The listing builds one solid part. Answer for the finished solid, in the listing's coordinates (mm). A direction names the side the tool comes from. Coordinates: 2 decimals unless noted, no trailing zeros. Write each loop counter-clockwise with the first axis right and the second up, starting at its lowest first coordinate (ties: lowest second). Pieces come first, ordered by that corner, then holes.
Autodesk Inventor part; units mm, degrees
ref_plane "Arbeitsebene2" through (-22.5, -14.565, -0.4115) normal (0, 0, -1) x (0, 1, 0)
ref_plane "Arbeitsebene3" through (-22.5, -14.565, 0) normal (0, 0, 1) x (1, 0, 0)
ref_plane "YZ Plane" through (0, 0, 0) normal (1, 0, 0) x (0, 1, 0)
ref_plane "Arbeitsebene1" through (0, 0, 6) normal (0, 0, 1) x (1, 0, 0)
sketch "Skizze3" plane through (0, 0, 6) normal (0, 0, 1) x (1, 0, 0)
  line L0 (22.5, -14.565) -> (22.5, 14.565)
  line L1 (-22.5, -14.565) -> (22.5, -14.565)
  line L2 (-22.5, 10.565) -> (-22.5, -14.565)
  line L3 (22.5, 14.565) -> (-18.5, 14.565)
  circle A0 centre (19.6, -11.465) radius 1.5
  circle A1 centre (13.06, -2.125) radius 0.65
  circle A2 centre (13.06, -4.665) radius 0.65
  circle A3 centre (13.06, 0.415) radius 0.65
  circle A4 centre (13.06, 2.955) radius 0.65
  circle A5 centre (-2.18, 5.495) radius 0.65
  circle A6 centre (13.06, 5.495) radius 0.65
  circle A7 centre (19.6, 11.535) radius 1.5
  circle A8 centre (13.06, 8.035) radius 0.65
  circle A9 centre (13.06, 10.575) radius 0.65
  circle A10 centre (-2.18, 8.035) radius 0.65
  circle A11 centre (13.06, 13.115) radius 0.65
  circle A12 centre (-2.18, 10.575) radius 0.65
  circle A13 centre (-7.26, -6.945) radius 0.5
  circle A14 centre (-2.18, -2.125) radius 0.65
  circle A15 centre (-2.18, -4.665) radius 0.65
  circle A16 centre (-12.34, -6.945) radius 0.5
  circle A17 centre (-19.4, -11.465) radius 1.5
  circle A18 centre (-7.26, -4.405) radius 0.5
  circle A19 centre (-12.34, -4.405) radius 0.5
  circle A20 centre (-2.18, 0.415) radius 0.65
  circle A21 centre (-2.18, 13.115) radius 0.65
  circle A22 centre (-2.18, 2.955) radius 0.65
  circle A23 centre (-7.26, -1.865) radius 0.5
  circle A24 centre (-12.34, -1.865) radius 0.5
  circle A25 centre (-7.26, 0.675) radius 0.5
  circle A26 centre (-12.34, 0.675) radius 0.5
  line L4 (-24.7, -16.765) -> (24.7, -16.765)
  line L5 (24.7, -16.765) -> (24.7, 16.765)
  line L6 (24.7, 16.765) -> (-24.7, 16.765)
  line L7 (-24.7, 16.765) -> (-24.7, -16.765)
  line L8 (-24.34, 2.175) -> (-10.84, 2.175)
  line L9 (-10.84, 2.175) -> (-10.84, -8.525)
  line L10 (-10.84, -8.525) -> (-24.34, -8.525)
  line L11 (-24.34, -8.525) -> (-24.34, 2.175)
  circle A27 centre (-12.34, -1.865) radius 0.5
  circle A28 centre (-12.34, -4.405) radius 0.5
  circle A29 centre (-12.34, -6.945) radius 0.5
  circle A30 centre (-12.34, 0.675) radius 0.5
  circle A31 centre (-21.39, -0.725) radius 1.5
  line L12 (24.7, 16.765) -> (-26.94, 16.765)
  line L13 (-26.94, 16.765) -> (-26.94, -16.765)
  line L14 (-26.94, -16.765) -> (24.7, -16.765)
  line L15 (24.7, -16.765) -> (24.7, 16.765)
  line L16 (-18.5, 10.565) -> (-18.5, 14.565)
  line L17 (-22.5, 10.565) -> (-18.5, 10.565)
  point P0 (0, 0)
  point P1 (-24.7, 16.765)
  dimension "d5" = 2.2
  dimension "d6" = 2.6
extrude "Extrusion2" add sketch "Skizze3" against normal blind 2 contours L1 L2 L10 L9 L8 L17 L16 L3 L0 | L10 L11 L8 L2 A31 | L2 A31 L8 L9 L10 | A31 L2 | L2 A31 | A0 | A1 | A2 | A3 | A4 | A5 | A6 | A7 | A8 | A9 | A10 | A11 | A12 | A13 | A14 | A15 | A16 | A17 | A18 | A19 | A20 | A21 | A22 | A23 | A24 | A25 | A26 | L7 L6 L5 L4 | L14 L13 L12 L7
sketch "Skizze4" plane through (0, 0, 4) normal (0, 0, -1) x (-1, 0, 0)
  line L0 (-24.7, 16.765) -> (-24.7, -16.765)
  line L1 (-24.7, -16.765) -> (26.94, -16.765)
  line L2 (26.94, -16.765) -> (26.94, 16.765)
  line L3 (26.94, 16.765) -> (-24.7, 16.765)
  line L4 (-22.7, 14.765) -> (-22.7, -14.765)
  line L5 (-22.7, -14.765) -> (24.94, -14.765)
  line L6 (24.94, -14.765) -> (24.94, 14.765)
  line L7 (24.94, 14.765) -> (-22.7, 14.765)
  point P0 (0, 0)
  dimension "d9" = 2
ref_plane "Arbeitsebene2" through (-22.5, -14.565, -0.4115) normal (0, 0, -1) x (0, 1, 0)
extrude "Extrusion3" add sketch "Skizze4" along normal up to surface (4.4115 mm away)
sketch "Skizze5" plane through (24.7, -16.765, -0.4115) normal (0, 0, -1) x (-1, 0, 0)
  line L0 (2, 31.53) -> (2, 2)
  line L1 (49.64, 31.53) -> (2, 31.53)
  line L2 (49.64, 2) -> (49.64, 31.53)
  line L3 (2, 2) -> (49.64, 2)
  line L4 (0, 0) -> (0, 33.53)
  line L5 (51.64, 0) -> (0, 0)
  line L6 (51.64, 33.53) -> (51.64, 0)
  line L7 (0, 33.53) -> (51.64, 33.53)
  line L8 (50.64, 32.53) -> (50.64, 1)
  line L9 (50.64, 1) -> (1, 1)
  line L10 (1, 1) -> (1, 32.53)
  line L11 (1, 32.53) -> (50.64, 32.53)
  point P0 (24.7, 16.765)
  dimension "d12" = 1
extrude "Extrusion4" cut sketch "Skizze5" against normal blind 2 contours L4 L7 L6 L5
sketch "Skizze6" plane through (0, 0, 4) normal (0, 0, -1) x (-1, 0, 0)
  circle A0 centre (-19.6, 11.535) radius 1.5
  circle A1 centre (-19.6, -11.465) radius 1.5
  circle A2 centre (19.4, -11.465) radius 1.5
  circle A3 centre (-19.6, -11.465) radius 1.7
  circle A4 centre (-19.6, 11.535) radius 1.7
  circle A5 centre (19.4, -11.465) radius 1.7
  line L0 (-22.7, -14.765) -> (24.94, -14.765)
  line L1 (-22.7, -14.765) -> (-16.5, -14.765)
  line L2 (-16.5, -14.765) -> (-16.5, -10.165)
  line L3 (-18.5, -8.165) -> (-22.7, -8.165)
  line L4 (-22.7, -8.165) -> (-22.7, -14.765)
  arc A6 (-16.5, -10.165) -> (-18.5, -8.165) centre (-18.5, -10.165) ccw
  line L5 (24.94, 14.765) -> (-22.7, 14.765)
  line L6 (-22.7, 14.765) -> (-16.5, 14.765)
  line L7 (-16.5, 14.765) -> (-16.5, 10.165)
  line L8 (-18.5, 8.165) -> (-22.7, 8.165)
  line L9 (-22.7, 8.165) -> (-22.7, 14.765)
  line L10 (24.94, -14.765) -> (16.3, -14.765)
  line L11 (16.3, -14.765) -> (16.3, -10.165)
  line L12 (18.3, -8.165) -> (24.94, -8.165)
  line L13 (24.94, -8.165) -> (24.94, -14.765)
  arc A7 (18.3, -8.165) -> (16.3, -10.165) centre (18.3, -10.165) ccw
  arc A8 (-18.5, 8.165) -> (-16.5, 10.165) centre (-18.5, 10.165) ccw
  line L14 (24.94, 14.765) -> (16.3, 14.765)
  line L15 (16.3, 14.765) -> (16.3, 10.165)
  line L16 (18.3, 8.165) -> (24.94, 8.165)
  line L17 (24.94, 8.165) -> (24.94, 14.765)
  arc A9 (16.3, 10.165) -> (18.3, 8.165) centre (18.3, 10.165) ccw
  point P0 (0, 0)
  point P1 (-16.5, -8.165)
  point P2 (-16.5, 8.165)
  dimension "d15" = 0.2
  dimension "d16" = 0.2
  dimension "d17" = 0.2
  dimension "d18" = 6.2
  dimension "d19" = 6.6
  dimension "d20" = 2
  dimension "d21" = 6.2
  dimension "d22" = 6.6
  dimension "d23" = 3.3
  dimension "d24" = 3.1
  dimension "d25" = 2
  dimension "d26" = 2
ref_plane "Arbeitsebene3" through (-22.5, -14.565, 0) normal (0, 0, 1) x (1, 0, 0)
extrude "Extrusion5" add sketch "Skizze6" along normal blind 2.211 contours L4 L3 A6 L2 L0 | L11 A7 L12 L13 L0 | L17 L16 A9 L15 L5 | L7 A8 L8 L9 L5
sketch "Skizze7" plane through (19.6, 11.535, 4) normal (0, 0, -1) x (-1, 0, 0)
  circle A0 centre (0, 0) radius 1.7
  circle A1 centre (0, -23) radius 1.7
  circle A2 centre (39, -23) radius 1.7
  point P0 (19.6, -11.535)
extrude "Extrusion6" cut sketch "Skizze7" against normal up to surface (2 mm away)
sketch "Skizze8" plane through (0, 0, 6) normal (0, 0, 1) x (1, 0, 0)
  circle A0 centre (19.6, -11.465) radius 1.7
  circle A1 centre (19.6, 11.535) radius 1.7
  circle A2 centre (-19.4, -11.465) radius 1.7
  line L0 (24.7, -16.765) -> (24.7, 16.765)
  line L1 (24.7, 16.765) -> (-26.94, 16.765)
  line L2 (-26.94, 16.765) -> (-26.94, -16.765)
  line L3 (-26.94, -16.765) -> (24.7, -16.765)
  line L4 (16.75, -9.8196) -> (19.6, -8.1741)
  line L5 (19.6, -8.1741) -> (22.45, -9.8196)
  line L6 (22.45, -9.8196) -> (22.45, -13.1104)
  line L7 (22.45, -13.1104) -> (19.6, -14.7559)
  line L8 (19.6, -14.7559) -> (16.75, -13.1104)
  line L9 (16.75, -13.1104) -> (16.75, -9.8196)
  line L10 (16.75, 13.1804) -> (19.6, 14.8259)
  line L11 (19.6, 14.8259) -> (22.45, 13.1804)
  line L12 (22.45, 13.1804) -> (22.45, 9.8896)
  line L13 (22.45, 9.8896) -> (19.6, 8.2441)
  line L14 (19.6, 8.2441) -> (16.75, 9.8896)
  line L15 (16.75, 9.8896) -> (16.75, 13.1804)
  line L16 (-22.25, -9.8196) -> (-19.4, -8.1741)
  line L17 (-19.4, -8.1741) -> (-16.55, -9.8196)
  line L18 (-16.55, -9.8196) -> (-16.55, -13.1104)
  line L19 (-16.55, -13.1104) -> (-19.4, -14.7559)
  line L20 (-19.4, -14.7559) -> (-22.25, -13.1104)
  line L21 (-22.25, -13.1104) -> (-22.25, -9.8196)
  line L22 (24.7, -16.765) -> (24.7, 16.765)
  point P0 (0, 0)
  dimension "d31" = 5.7
  dimension "d32" = 5.7
  dimension "d33" = 5.7
extrude "Extrusion7" cut sketch "Skizze8" against normal blind 2.6 contours A0 | A1 | A2 | L4 L5 L6 L7 L8 L9 | L10 L11 L12 L13 L14 L15 | L16 L17 L18 L19 L20 L21
fillet "Rundung1" radius 2 4 edges at (24.7, -16.765, 3.7943) (-26.94, -16.765, 3.7943) (-26.94, 16.765, 5) (24.7, 16.765, 3.7943)
fillet "Rundung2" radius 1 4 edges at (-25.94, -15.765, 0.5885) (-25.94, 15.765, 0.5885) (23.7, 15.765, 0.5885) (23.7, -15.765, 0.5885)
sketch "Skizze9" plane through (0, 0, 1.789) normal (0, 0, -1) x (-1, 0, 0)
  line L0 (24.94, 14.765) -> (24.94, 8.165)
  line L1 (24.94, 14.765) -> (21.64, 14.765)
  line L2 (21.64, 14.765) -> (21.64, 11.465)
  line L3 (21.64, 11.465) -> (24.94, 11.465)
  line L4 (24.94, 11.465) -> (24.94, 14.765)
  circle A0 centre (23.29, 13.115) radius 1.65
  point P0 (0, 0)
  dimension "d38" = 3.3
  dimension "d39" = 3.3
extrude "Extrusion8" cut sketch "Skizze9" against normal blind 10 contours A0
sketch "Skizze10" plane through (0, 0, 6) normal (0, 0, 1) x (1, 0, 0)
  arc A0 (-24.94, 13.115) -> (-23.29, 14.765) centre (-23.29, 13.115) ccw
  line L0 (-20.44, 11.4696) -> (-23.29, 9.8241)
  line L1 (-23.29, 9.8241) -> (-26.14, 11.4696)
  line L2 (-26.14, 11.4696) -> (-26.14, 14.7604)
  line L3 (-26.14, 14.7604) -> (-23.29, 16.4059)
  line L4 (-23.29, 16.4059) -> (-20.44, 14.7604)
  line L5 (-20.44, 14.7604) -> (-20.44, 11.4696)
  line L6 (-26.94, 14.765) -> (-26.94, -14.765)
  point P0 (0, 0)
  point P1 (-26.14, 13.115)
  dimension "d42" = 5.7
extrude "Extrusion9" cut sketch "Skizze10" against normal blind 2.6
properties part number "Gehaeuse_unten"
1. Flat-ended cylindrical pins translate along their axes: P1, Ø4, axis at x = 19.6, y = 11.535, coming from the -Z side; P2, Ø2, axis at x = -23.29, y = 13.115, coming from the -Z side; P3, Ø2, axis at y = 5, z = 0.5, coming from the +X side; P4, Ø0.6, axis at y = 1, z = 1, coming from the -X side. Find the tip coordinate at first contact, or state that the pin passes through.
Results found:
P1: stops at z = 1.79
P2: passes through
P3: stops at x = 23.7
P4: stops at x = -25.94
2. Section C-C on z = 0.75 is taken. Give the vertices of the cut face in (x, y) (3 decimals), then the cut area to 3 significant figures.
Results found:
outline: (-25.94, -14.765) arc R1 ccw to (-24.94, -15.765) - (22.7, -15.765) arc R1 ccw to (23.7, -14.765) - (23.7, 14.765) arc R1 ccw to (22.7, 15.765) - (-24.94, 15.765) arc R1 ccw to (-25.94, 14.765) - close; hole (-24.94, -14.765) - (22.7, -14.765) - (22.7, 14.765) - (-24.94, 14.765) - close
area: 157 mm2
3. A tool of negligible diameter and unlimited length cuts with its end or side. For faces 4 (the flat face through (-24.735, 15.572, 4.718)), 5 (the cylindrical face through (24.13, -16.164, 3.763)), 6 (the flat face through (22.7, 0, 1)), from which of +Z, -Z, +X, -X, +Y, -Y can it reach the whole face along a straight path? Write none if from no direction.
Results found:
face 4: +Z
face 5: +Z, -Z, +X, -Y
face 6: -Z
4. Find the intervals of material crossed by L1, parallel to Y at x = -19.4, z = 3.05 (3 decimals); L2, parallel to Y at x = 19.6, z = 2.25 (3 decimals); L3, parallel to X at y = -14.5, z = 2.25, in increasing order.
Results found:
L1: y = -16.765 to -13.165, -9.765 to -8.165, 8.165 to 16.765
L2: y = -16.765 to -13.165, -9.765 to -8.165, 8.165 to 9.835, 13.235 to 16.765
L3: x = -26.94 to -16.3, 16.5 to 24.7
5. Section A-A on z = 5.25 is taken. State how many separate pieces and enclosed holes the cut face has, then the cut area to 3 significant figures.
Results found:
separate pieces: 1
enclosed holes: 4
area: 1,620 mm2
6. For a pull along Y with two mould halves and no side action, classify faces 1 (the flat face through (-26.94, 0, 4)), 2 (the flat face through (-21.845, 10.658, 4.718)), 3 (the flat face through (-1, -15.765, 1)) as pulls with the +Y half, pulls with the -Y half, needs draft (parallel to the pull), parting line crosses it, or undercut.
Results found:
face 1: needs draft
face 2: undercut
face 3: pulls with the -Y half
7. Section B-B on x = 11.5 is taken. Give the vertices of the cut face in (y, z) (1 decimal).
Results found:
outline: (-16.8, 1.6) - (-15.8, 1.6) - (-15.8, -0.4) - (-14.8, -0.4) - (-14.8, 4) - (14.8, 4) - (14.8, -0.4) - (15.8, -0.4) - (15.8, 1.6) - (16.8, 1.6) - (16.8, 6) - (-16.8, 6) - close
8. Section D-D on y = 3 is taken. Give the vertices of the cut face in (x, z).
Results found:
outline: (-26.94, 1.59) - (-25.94, 1.59) - (-25.94, -0.41) - (-24.94, -0.41) - (-24.94, 4) - (22.7, 4) - (22.7, -0.41) - (23.7, -0.41) - (23.7, 1.59) - (24.7, 1.59) - (24.7, 6) - (-26.94, 6) - close
